Source: CAD feature listing. Evaluate the final solid. Frame: model axes, mm. Give positions to 0.01 mm unless a question says otherwise; leave off trailing zeros. Order: outer loops, then holes, each group sorted by start corner. A loop starts at its lowest first (then second) coordinate and runs counter-clockwise, first axis right, second up. Notation, with made-up numbers: (19, -35) - (51, -35) arc R28 ccw to (51, -9) - close; hole circle Ø2 at (80, 31.25). An arc over 180 degrees is marked (long way). Answer as CSV lines item,"result".
```python
from build123d import *

# Parameters (mm, degrees)
SKETCH2_R           = 1.5
BOSS_EXTRUDE1_DEPTH = 1.25
CHAMFER1_SIZE       = 0.25


with BuildPart() as part:
    # Sketch2 → Boss-Extrude1 (new, symmetric)
    with BuildSketch(Plane(origin=(0, 0, 0), x_dir=(1, 0, 0), z_dir=(0, 1, 0))):
        Polygon((-2.725, 1.573279484), (-2.725, -1.573279484), (0, -3.146558967), (2.725, -1.573279484), (2.725, 1.573279484), (0, 3.146558967), align=None)
        with Locations(Location((0, 0, 0), (0, 0, 270))):
            Circle(SKETCH2_R, mode=Mode.SUBTRACT)
    extrude(amount=BOSS_EXTRUDE1_DEPTH, both=True)

    # Chamfer1
    chamfer1_edges = [part.edges().sort_by_distance(p)[0] for p in [
        (0, -1.25, -1.5),
        (0, 1.25, -1.5),
    ]]
    chamfer(chamfer1_edges, length=CHAMFER1_SIZE)


solid = part.part
```
(1) Cut plane C-C (x = 2.15). Return loops of the section in (y, z), then the cut area to 3 significant figures.
Completed:
outline,"(-1.25, -1.91) - (1.25, -1.91) - (1.25, 1.91) - (-1.25, 1.91) - close"
area,"9.53 mm²"
(2) Ray query, line 1 (X direction, y = -0.4, z = 0) (3 decimals); line 2 (Z direction, x = -1.2, y = -0.1); line 3 (Z direction, x = 0.5, y = -0.9). Return the intervals inside material, ascending. Write a range as from..to.
Completed:
line 1,"-2.725..-1.5, 1.5..2.725"
line 2,"-2.45..-0.9, 0.9..2.45"
line 3,"-2.86..-1.41, 1.41..2.86"
(3) Cut plane A-A (z = 0). Return loops of the section in (x, y) (3 decimals), then the cut area to 3 significant figures.
Completed:
outline,"(-2.725, -1.25) - (-1.75, -1.25) - (-1.5, -1) - (-1.5, 1) - (-1.75, 1.25) - (-2.725, 1.25) - close; (1.5, -1) - (1.75, -1.25) - (2.725, -1.25) - (2.725, 1.25) - (1.75, 1.25) - (1.5, 1) - close"
area,"6.00 mm²"
(4) Cut plane B-B (y = 0.55). Return loops of the section in (x, z) (3 decimals), then the cut area to 3 significant figures.
Completed:
outline,"(-2.725, -1.573) - (0, -3.147) - (2.725, -1.573) - (2.725, 1.573) - (0, 3.147) - (-2.725, 1.573) - close; hole circle Ø3 at (0, 0)"
area,"18.7 mm²"
(5) Cut plane D-D (z = 2). Return loops of the section in (x, y), then the cut area to 3 significant figures.
Completed:
outline,"(-1.99, -1.25) - (1.99, -1.25) - (1.99, 1.25) - (-1.99, 1.25) - close"
area,"9.93 mm²"
(6) Mould query, pull axis X, two halves, no side actions, for faces 1 (the cylindrical face through (0.45, -0.01, 1.43)), 2 (the flat face through (-1.38, 0.02, 2.35)), 3 (the flat face through (1.38, 0.02, -2.35)), 4 (the flat face through (-2, -1.25, 0)). Classes: released by +X, released by -X, zero draft, split by the parting line, or undercut.
Completed:
face 1,"undercut"
face 2,"released by -X"
face 3,"released by +X"
face 4,"zero draft"
(7) Contact query for flat-ended pins moving along their axis: pin 1 (1 mm diameter, centred on x = 1, y = 0.5, fed in from -Z); pin 2 (1 mm diameter, centred on x = 2, y = -0.5, fed in from +Z). Output: stop coordinate, or through.
Completed:
pin 1,"z = -2.86"
pin 2,"z = 2.28"
